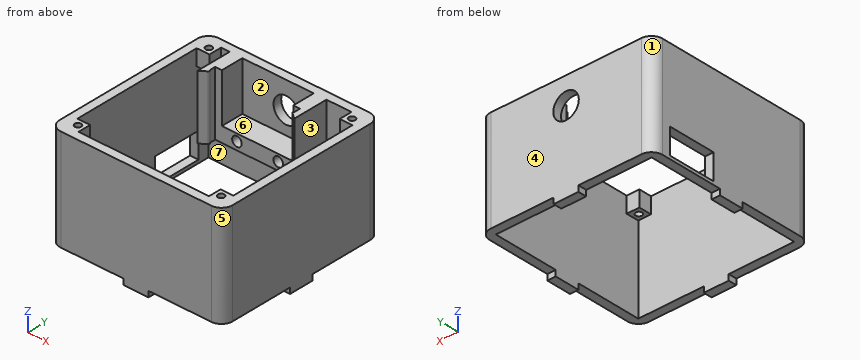
Autodesk Inventor part; units mm, degrees
ref_plane "Arbeitsebene1" through (-2.592, 17.461, 16.63) normal (1, 0, 0) x (0, 0, -1)
ref_plane "YZ Plane" through (0, 0, 0) normal (1, 0, 0) x (0, 1, 0)
ref_plane "XZ Plane" through (0, 0, 0) normal (0, 1, 0) x (-1, 0, 0)
sketch "Skizze1" plane through (0, 0, 0) normal (0, 0, 1) x (1, 0, 0)
  line L0 (-27.13, -27.13) -> (27.13, -27.13)
  line L1 (27.13, -27.13) -> (27.13, 27.13)
  line L2 (27.13, 27.13) -> (-27.13, 27.13)
  line L3 (-27.13, 27.13) -> (-27.13, -27.13)
  line L4 (-37.982, 0) -> (37.982, 0) construction
  line L5 (0, -37.982) -> (0, 37.982) construction
  line L6 (-24.484, 24.484) -> (24.484, 24.484)
  line L7 (24.484, 24.484) -> (24.484, -24.484)
  line L8 (24.484, -24.484) -> (-24.484, -24.484)
  line L9 (-24.484, -24.484) -> (-24.484, 24.484)
  point P0 (0, 0)
  dimension "d0" = 54.26
  dimension "d1" = 2.646
extrude "Extrusion1" add sketch "Skizze1" along normal blind 32
fillet "Rundung1" radius 3.5 4 edges at (-27.13, 27.13, 16) (27.13, 27.13, 16) (-27.13, -27.13, 16) (27.13, -27.13, 16)
sketch "Skizze2" plane through (0, 0, 32) normal (0, 0, 1) x (1, 0, 0)
  line L0 (-24.484, -24.484) -> (-24.484, 24.484)
  line L1 (-24.484, 24.484) -> (24.484, 24.484)
  line L2 (-24.484, 20.484) -> (-20.484, 20.484)
  line L3 (-20.484, 20.484) -> (-20.484, 24.484)
  line L4 (-20.484, 24.484) -> (-24.484, 24.484)
  line L5 (-24.484, 24.484) -> (-24.484, 20.484)
  point P0 (0, 0)
  point P1 (-24.484, 20.984)
  point P2 (-20.984, 24.484)
  point P3 (20.984, 24.484)
  point P4 (-24.484, 20.984)
  point P5 (-20.984, 24.484)
  dimension "d5" = 4
extrude "Extrusion2" add sketch "Skizze2" against normal blind 5
sketch "Skizze3" plane through (0, 0, 32) normal (0, 0, 1) x (1, 0, 0)
  line L0 (-24.484, 20.484) -> (-20.484, 20.484)
  line L1 (-20.484, 20.484) -> (-20.484, 24.484)
  point P0 (0, 0)
  point P1 (-22.484, 22.484)
  dimension "d8" = 2
  dimension "d9" = 2
hole "Bohrung1" at (-22.484, 22.484, 32) direction (0, 0, -1) diameter 2 depth 5
pattern_circular "Runde Anordnung1" count 4 over 360 about axis through (0, 0, -10) along (0, 0, 1) of "Extrusion2", "Bohrung1"
sketch "Skizze4" plane through (-20.984, 24.484, 0) normal (0, -1, 0) x (1, 0, 0)
  line L0 (41.468, 27) -> (41.468, 32)
  line L1 (0.5, 32) -> (41.468, 32)
  line L2 (0.5, 32) -> (0.5, 27)
  line L3 (0.5, 27) -> (-3.5, 27)
  line L4 (-3.5, 0) -> (45.468, 0)
  line L5 (45.468, 27) -> (41.468, 27)
  line L6 (44.614, 32) -> (-2.646, 32)
  line L7 (3.184, 32) -> (7.184, 32)
  line L8 (7.184, 32) -> (7.184, 11.949)
  line L9 (7.184, 11.949) -> (3.184, 11.949)
  line L10 (3.184, 11.949) -> (3.184, 32)
  line L11 (7.184, 11.949) -> (29.6, 11.949)
  line L12 (29.6, 11.949) -> (29.6, 16.63)
  line L13 (29.6, 16.63) -> (7.184, 16.63)
  line L14 (7.184, 16.63) -> (7.184, 11.949)
  line L15 (0.5, 32) -> (41.468, 32)
  line L16 (29.6, 11.949) -> (33.6, 11.949)
  line L17 (33.6, 11.949) -> (33.6, 32)
  line L18 (33.6, 32) -> (29.6, 32)
  line L19 (29.6, 32) -> (29.6, 11.949)
  line L20 (-3.5, 0) -> (-3.5, 27)
  line L21 (45.468, 0) -> (45.468, 27)
  point P0 (20.984, 0)
  point P1 (18.392, 11.949)
  point P2 (33.6, 32)
  point P3 (7.184, 16.63)
  dimension "d20" = 4
  dimension "d21" = 4.681
  dimension "d22" = 22.416
  dimension "d23" = 2.684
  dimension "d24" = 15.37
extrude "Extrusion3" add sketch "Skizze4" along normal blind 7.023 contours L17 L16 L12 L19 L1 | L8 L9 L10 L1 | L12 L11 L8 L13
sketch "Skizze5" plane through (0, 0, 32) normal (0, 0, 1) x (1, 0, 0)
  line L0 (-17.8, 17.461) -> (12.616, 17.461)
  line L1 (-17.8, 17.461) -> (-15.9, 17.461)
  line L2 (-17.8, 15.0145) -> (-17.8, 17.461)
  line L3 (-17.8, 15.0145) -> (-17.8, 13.484)
  line L4 (-17.8, 13.484) -> (-15.806, 14.94)
  line L5 (-20.484, 24.484) -> (-17.8, 24.484)
  arc A0 (-15.806, 14.94) -> (-15.9, 15.637) centre (-16.0419, 15.263) ccw
  line L6 (-15.9, 15.637) -> (-15.9, 17.461)
  point P0 (0, 0)
  dimension "d27" = 11
  dimension "d30" = 0.4
  dimension "d31" = 1.824
  dimension "d32" = 1.9
  dimension "d33" = 1.994
extrude "Extrusion4" add sketch "Skizze5" against normal up to surface (20.051 mm away)
ref_plane "Arbeitsebene1" through (-2.592, 17.461, 16.63) normal (1, 0, 0) x (0, 0, -1)
sketch "Skizze7" plane through (-20.984, 17.461, 0) normal (0, -1, 0) x (1, 0, 0)
  line L0 (33.6, 32) -> (29.6, 32)
  line L1 (29.6, 32) -> (29.6, 16.63)
  line L2 (29.6, 16.63) -> (7.184, 16.63)
  line L3 (7.184, 16.63) -> (7.184, 32)
  line L4 (7.184, 32) -> (5.084, 32)
  line L5 (5.084, 32) -> (5.084, 11.949)
  line L6 (5.084, 11.949) -> (33.6, 11.949)
  line L7 (33.6, 11.949) -> (33.6, 32)
  point P0 (20.984, 0)
  point P1 (11.915, 14.413)
  dimension "d36" = 2.464
  dimension "d37" = 4.731
hole "Bohrung2" at (-9.069, 17.461, 14.413) direction (0, 1, 0) diameter 3 depth 7.023
mirror "Spiegeln2" about plane through (-2.592, 17.461, 16.63) normal (1, 0, 0) of "Extrusion4", "Bohrung2"
sketch "Skizze8" plane through (-23.63, 27.13, 0) normal (0, 1, 0) x (1, 0, 0)
  line L0 (47.26, -32) -> (0, -32)
  line L1 (23.63, -32) -> (23.63, 0) construction
  point P0 (23.63, -23.607)
  dimension "d45" = 8.393
hole "Bohrung3" at (0, 27.13, 23.607) direction (0, -1, 0) diameter 8 depth 2.646
sketch "Skizze9" plane through (0, 0, 0) normal (0, 0, -1) x (-1, 0, 0)
  line L0 (-23.63, 27.13) -> (23.63, 27.13)
  line L1 (13.8, 24.484) -> (-8.616, 24.484)
  line L2 (-3.9, 27.13) -> (3.9, 27.13)
  line L3 (3.9, 27.13) -> (3.9, 24.484)
  line L4 (3.9, 24.484) -> (-3.9, 24.484)
  line L5 (-3.9, 24.484) -> (-3.9, 27.13)
  line L6 (0, -37.982) -> (0, 37.982) construction
  point P0 (0, 0)
  dimension "d53" = 7.8
extrude "Extrusion5" add sketch "Skizze9" along normal blind 1.8
pattern_circular "Runde Anordnung2" count 4 over 360 about axis through (0, 0, -10) along (0, 0, 1) of "Extrusion5"
sketch "Skizze10" plane through (-27.13, -23.63, 32) normal (-1, 0, 0) x (0, 0, 1)
  line L0 (-23, 44.76) -> (-31, 44.76)
  line L1 (-31, 44.76) -> (-31, 29.76)
  line L2 (-31, 29.76) -> (-23, 29.76)
  line L3 (-23, 29.76) -> (-23, 44.76)
  line L4 (0, 50.76) -> (-32, 50.76)
  line L5 (-32, 47.26) -> (-32, 27.53)
  point P0 (-32, 23.63)
  dimension "d59" = 6
  dimension "d60" = 8
  dimension "d61" = 15
  dimension "d62" = 1
extrude "Extrusion6" cut sketch "Skizze10" against normal up to surface (2.646 mm away)
properties part number "brick_shell_+USB_nudge_V3"
Verification items for the finished model (mm, model axes). Face numbers are marked on the shaded views. A direction names the side the tool comes from. Give positions to 0.01 mm unless a question says otherwise; leave off trailing zeros. Order: outer loops, then holes, each group sorted by start corner. A loop starts at its lowest first (then second) coordinate and runs counter-clockwise, first axis right, second up. Notation, with made-up numbers: (49.5, 49.25) -> (99.5, 49.25) arc R16 cw to (99.5, 63.25) -> close; hole circle Ø9 at (-14, -25.75). An arc over 180 degrees is marked (long way). Use a Markdown table: item, result.
1) Section check C-C, the plane x = -12. Record the boundary of the cut face in (y, z).
Results:
| item | result |
|---|---|
| outline | (-27.13, 0) -> (-24.48, 0) -> (-24.48, 32) -> (-27.13, 32) -> close; (17.46, 11.95) -> (24.48, 11.95) -> (24.48, 0) -> (27.13, 0) -> (27.13, 32) -> (24.48, 32) -> (24.48, 16.63) -> (17.46, 16.63) -> close |
2) Section check A-A, the plane y = -12. Record the boundary of the cut face in (x, z), then the cut area to 3 significant figures.
Results:
| item | result |
|---|---|
| outline | (-27.13, 0) -> (-24.48, 0) -> (-24.48, 32) -> (-27.13, 32) -> close; (24.48, 0) -> (27.13, 0) -> (27.13, 32) -> (24.48, 32) -> close |
| area | 169 mm² |
3) Tool access check on the marked faces 5, 6 and 7. Record the directions out of +Z, -Z, +X, -X, +Y, -Y that give a thin tool (end or side, any length) a straight path to the whole face; none if there is none.
Results:
| item | result |
|---|---|
| face 5 | +Z, -Z, +X, -Y |
| face 6 | +Z |
| face 7 | -Z |
4) Mould release check, pull along X, two halves, no side actions. Record for the marked faces 1, 2, 3 and 4: pulls with the +X half, pulls with the -X half, needs draft (parallel to the pull), parting line crosses it, or undercut.
Results:
| item | result |
|---|---|
| face 1 | pulls with the -X half |
| face 2 | undercut |
| face 3 | undercut |
| face 4 | needs draft |
5) Material ranges on probe 1 along X at (y, z) = (19, 24); probe 2 along X at (y, z) = (-19, 16.5); probe 3 along X at (y, z) = (15, 20), recorded low to high.
Results:
| item | result |
|---|---|
| probe 1 | -27.13 to -24.48, -17.8 to -13.8, 8.62 to 12.62, 24.48 to 27.13 |
| probe 2 | -27.13 to -24.48, 24.48 to 27.13 |
| probe 3 | -27.13 to -24.48, -17.8 to -15.74, 10.56 to 12.62, 24.48 to 27.13 |
6) Section check B-B, the plane x = 0. Record the boundary of the cut face in (y, z).
Results:
| item | result |
|---|---|
| outline | (-27.13, -1.8) -> (-24.48, -1.8) -> (-24.48, 32) -> (-27.13, 32) -> close; (17.46, 11.95) -> (24.48, 11.95) -> (24.48, -1.8) -> (27.13, -1.8) -> (27.13, 19.61) -> (24.48, 19.61) -> (24.48, 16.63) -> (17.46, 16.63) -> close; (24.48, 27.61) -> (27.13, 27.61) -> (27.13, 32) -> (24.48, 32) -> close |
7) Depth check by flat-ended pin: pin 1 Ø2 at (x, y) = (-21.5, -22) entering from -Z; pin 2 Ø1.4 at (x, z) = (25.5, -1) entering from +Y; pin 3 Ø1.8 at (x, y) = (22.484, -22.484) entering from -Z; pin 4 Ø5 at (x, y) = (2, 21.5) entering from +Z. Enter the tip coordinate at first touch or a pass-through.
Results:
| item | result |
|---|---|
| pin 1 | z = 27 |
| pin 2 | y = 3.9 |
| pin 3 | through |
| pin 4 | z = 16.63 |
